Read the model definition and answer for the solid it produces. Units are mm, in the model's axes. Face numbers are marked on the shaded views. A direction names the side the tool comes from. Round coordinates to 2 decimals unless told otherwise and drop trailing zeros. Write each loop counter-clockwise with the first axis right and the second up, starting at its lowest first coordinate (ties: lowest second). Pieces come first, ordered by that corner, then holes. Notation, with made-up numbers: (52, 64) -> (83, 64) arc R28 cw to (83, 84) -> close; hole circle Ø9 at (-5.75, 62). An arc over 180 degrees is marked (long way). Return JSON: item names as keys, results as strings.
from build123d import *

# Parameters (mm, degrees)
BOSS_EXTRUDE1_DEPTH = 13
FILLET1_R           = 0.8


with BuildPart() as part:
    # Sketch1 → Boss-Extrude1 (new body)
    with BuildSketch(Plane(origin=(0, 0, 0), x_dir=(1, 0, 0), z_dir=(0, 1, 0))):
        with BuildLine():
            Line((0, 51.7), (0, 53))
            ThreePointArc((0, 53), (-4, 49), (0, 45))
            ThreePointArc((0, 45), (40.783850417, 19.017821778), (34.47199994, -28.925442436))
            ThreePointArc((34.47199994, -28.925442436), (35.211540941, -37.378434753), (43.664533258, -36.638893752))
            Line((43.664533258, -36.638893752), (37.536177713, -31.496592875))
            ThreePointArc((37.536177713, -31.496592875), (48.870327604, -3.562454189), (41.707047143, 25.720074234))
            ThreePointArc((41.707047143, 25.720074234), (25.051905135, 42.111780407), (2.698975076, 48.925612245))
            ThreePointArc((2.698975076, 48.925612245), (-1.935309657, 47.117295421), (0, 51.7))
        make_face()
        with BuildLine():
            Line((51.921017872, 32.018867925), (0, 53))
            Line((0, 53), (0, 51.7))
            ThreePointArc((0, 51.7), (1.909188309, 50.909188309), (2.7, 49))
            ThreePointArc((2.7, 49), (2.699743757, 48.962802592), (2.698975076, 48.925612245))
            ThreePointArc((2.698975076, 48.925612245), (25.051905135, 42.111780407), (41.707047143, 25.720074234))
            Line((41.707047143, 25.720074234), (51.921017872, 32.018867925))
        make_face()
    extrude(amount=BOSS_EXTRUDE1_DEPTH)

    # Fillet1
    fillet1_edges = [part.edges().sort_by_distance(p)[0] for p in [
        (0, 6.5, -53),
        (51.921017872, 6.5, -32.018867925),
        (41.707047143, 6.5, -25.720074234),
        (37.536177713, 6.5, 31.496592875),
        (43.664533258, 6.5, 36.638893752),
    ]]
    fillet(fillet1_edges, radius=FILLET1_R)


solid = part.part
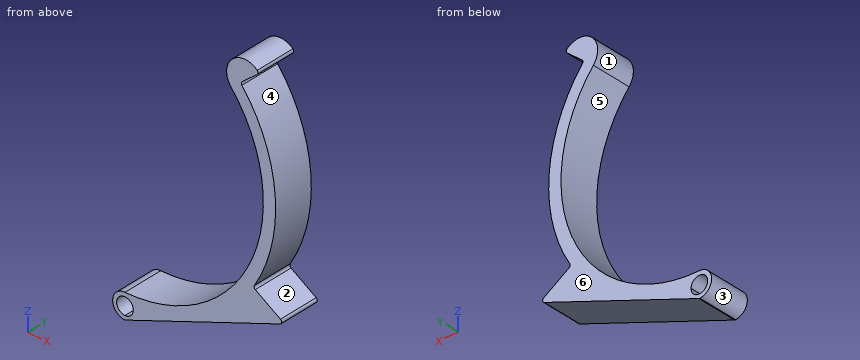
Item 1: Straight lines are drawn through the part: L1, parallel to Z at x = 0, y = 8; L2, parallel to Z at x = 38.5, y = 9.5; L3, parallel to Z at x = 41, y = 1. For each, find the intervals that lie inside material, in ascending order. Write a range as [from, to].
Worked answers:
{"L1": "z = [-52.98, -51.7], [-46.3, -45]", "L2": "z = [-37.44, -23.3], [23.3, 30.31], [32.31, 38.76]", "L3": "z = [-36.43, -18.55], [18.55, 26.83], [34.4, 38.46]"}
Item 2: Section B-B (x = 36.5) is taken. Give the vertices of the cut face in (y, z).
Worked answers:
{"outline": "(0, -38.25) -> (13, -38.25) -> (13, -26.32) -> (0, -26.32) -> close; (0, 26.32) -> (13, 26.32) -> (13, 38.2) -> (0, 38.2) -> close"}
Item 3: Section A-A (y = 8) is taken. Give the vertices of the cut face in (x, z).
Worked answers:
{"outline": "(-0.18, -53) arc R0.8 ccw to (0.15, -52.94) -> (50.45, -32.61) arc R0.8 ccw to (50.57, -31.19) -> (42.38, -26.14) arc R0.8 cw to (42.11, -25.05) arc R49 ccw to (38.04, 30.89) arc R0.8 cw to (38.14, 32.01) -> (43, 36.08) arc R0.8 ccw to (43.02, 37.3) arc R6 ccw to (34.47, 28.93) arc R45 cw to (0, -45) arc R4 ccw to start; hole (2.7, -49) arc R2.7 ccw to (2.7, -48.93) arc R2.7 ccw (long way) to start"}
Item 4: For a pull along Z with two mould halves and no side action, classify the marked faces 3, 4, 5 and 6 as released by +Z, released by -Z, zero draft, split by the parting line, or undercut.
Worked answers:
{"face 3": "split by the parting line", "face 4": "undercut", "face 5": "undercut", "face 6": "zero draft"}
Item 5: Section C-C (z = -10) is taken. Give the vertices of the cut face in (x, y).
Worked answers:
{"outline": "(43.87, 0) -> (47.97, 0) -> (47.97, 13) -> (43.87, 13) -> close"}
Item 6: Flat-ended cylindrical pins translate along their axes: pin 1 (1 mm diameter, centred on y = 6, z = 16.5, fed in from +X); pin 2 (4.5 mm diameter, centred on x = 0, z = -49, fed in from -Y); pin 3 (2 mm diameter, centred on x = 17.5, y = 3, fed in from +Z); pin 4 (5 mm diameter, centred on y = 10.5, z = -28.5, fed in from +X). Find the tip coordinate at first contact, or state that the pin passes through.
Worked answers:
{"pin 1": "stops at x = 46.31", "pin 2": "passes through", "pin 3": "stops at z = -41.02", "pin 4": "stops at x = 50.27"}
Item 7: Section D-D (x = 9) is taken. Give the vertices of the cut face in (y, z), then the cut area to 3 significant figures.
Worked answers:
{"outline": "(0, -49.36) -> (13, -49.36) -> (13, -44.09) -> (0, -44.09) -> close", "area": "68.5 mm2"}
Item 8: A tool of negligible diameter and unlimited length cuts with its end or side. For the marked faces 1 and 2, from which of +Z, -Z, +X, -X, +Y, -Y can it reach the whole face along a straight path? Write none if from no direction.
Worked answers:
{"face 1": "+Y, -Y", "face 2": "+X, +Y, -Y"}
